Can you work these out from the drawing? Everything is in mm from the part's minimum corner. Give positions to 0.01 mm unless a question says otherwise; leave off trailing zeros. Write each loop counter-clockwise with the first axis right and the second up, starting at its lowest first coordinate (ties: lowest second). Pieces come first, ordered by that corner, then holes. Notation, with made-up numbers: (-38, 66.5) -> (11, 66.5) arc R27 ccw to (11, 101.5) -> close; hole circle Ø1 at (-12.5, 53). An arc over 180 degrees is marked (long way). Return JSON: item names as keys, results as strings.
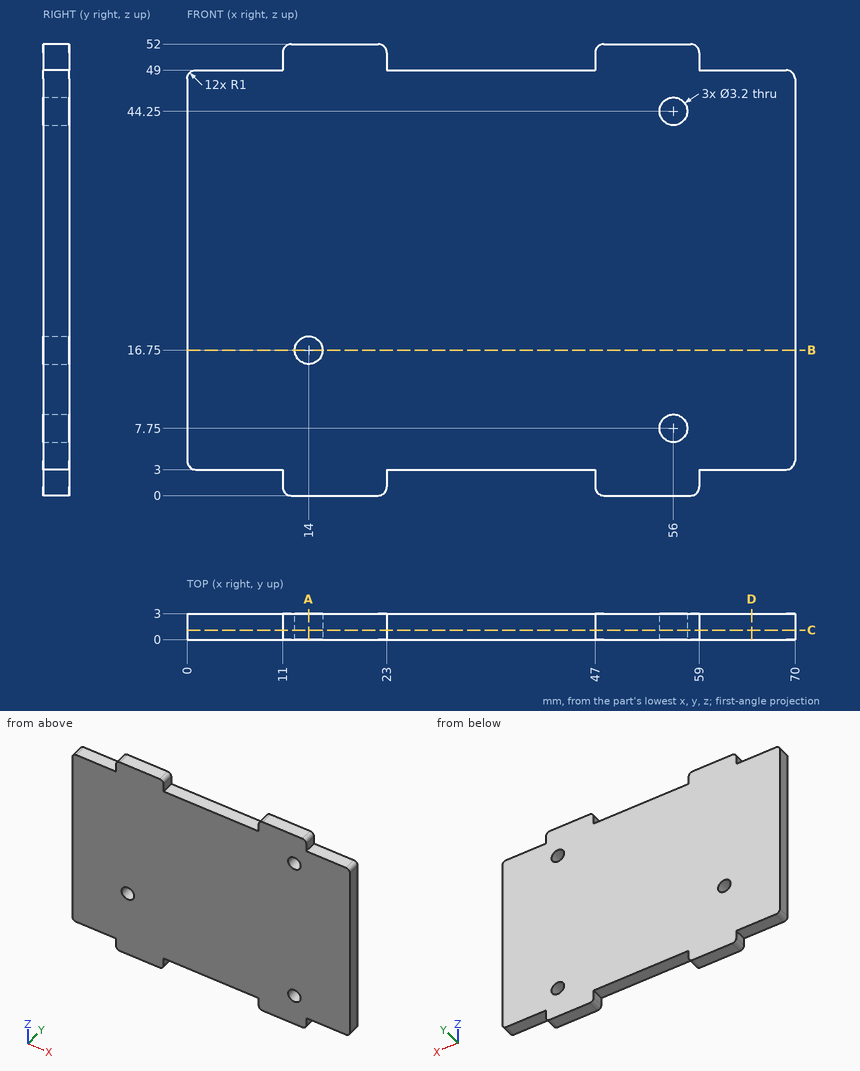
1. Suppose I cut it at C-C, the plane y = 1.1. Count the separate pieces of the cut face and the enclosed holes in it, and give its area (3 significant figures).
Taken from the geometry:
{"separate pieces": "1", "enclosed holes": "3", "area": "3,340 mm²"}
2. If I drill on line 1 (Z direction, x = 56, y = 2.4); line 2 (X direction, y = 1.15, z = 7.75); line 3 (X direction, y = 0.8, z = 43), over which ranges is the centre line in solid material (lowest first)? Write a range as [from, to].
Taken from the geometry:
{"line 1": "z = [0, 6.15], [9.35, 42.65], [45.85, 52]", "line 2": "x = [0, 54.4], [57.6, 70]", "line 3": "x = [0, 55], [57, 70]"}
3. Suppose I cut it at D-D, the plane x = 65. List the corners of the cut face in (y, z) for me, and give its area (3 significant figures).
Taken from the geometry:
{"outline": "(0, 3) -> (3, 3) -> (3, 49) -> (0, 49) -> close", "area": "138 mm²"}
4. Suppose I cut it at A-A, the plane x = 14. List the corners of the cut face in (y, z) for me, and give its area (3 significant figures).
Taken from the geometry:
{"outline": "(0, 0) -> (3, 0) -> (3, 15.15) -> (0, 15.15) -> close; (0, 18.35) -> (3, 18.35) -> (3, 52) -> (0, 52) -> close", "area": "146 mm²"}
5. For pin 1 Ø0.6 at (y, z) = (1, 50) entering from -X; pin 2 Ø1 at (x, y) = (9.5, 1.5) entering from -Z; pin 3 Ø2.5 at (x, z) = (14, 16.75) entering from -Y; pin 4 Ø0.6 at (y, z) = (1, 1.5) entering from +X, each with a flat end and sliding along its axis, tell me the tip position at first contact or that it passes through.
Taken from the geometry:
{"pin 1": "stops at x = 11", "pin 2": "stops at z = 3", "pin 3": "passes through", "pin 4": "stops at x = 59"}
6. Suppose I cut it at B-B, the plane z = 16.75. List the corners of the cut face in (x, y) for me.
Taken from the geometry:
{"outline": "(0, 0) -> (12.4, 0) -> (12.4, 3) -> (0, 3) -> close; (15.6, 0) -> (70, 0) -> (70, 3) -> (15.6, 3) -> close"}
